Work out the finished part from the listing and answer in its coordinate system (mm). A direction names the side the tool comes from. Coordinates: 2 decimals unless noted, no trailing zeros. Write each loop counter-clockwise with the first axis right and the second up, starting at its lowest first coordinate (ties: lowest second). Pieces come first, ordered by that corner, then holes. Notation, with made-up numbers: (25.25, 1) - (59.25, 1) arc R33 cw to (59.25, 30) - close; hole circle Ø10 at (32.25, 23.5). An arc over 180 degrees is marked (long way). Use one line per item in the form item = value. Start each with the question number.
Item 1: A cutting plane is placed at C-C (z = 1.7). Give the number of separate pieces and of enclosed holes in the cut face, then the cut area to 3 significant figures.
Item 2: A cutting plane is placed at A-A (x = 25). Write down the section's boundary in (y, z).
Item 3: Consider probe 1 along Y at (x, z) = (25, 2.45); probe 2 along X at (y, z) = (5.25, 1.85); probe 3 along X at (y, z) = (7, 2). Determine where each line is inside the solid, lowest interval first.
Item 4: A cutting plane is placed at D-D (y = 12). Write down the section's boundary in (x, z), then the cut area to 3 significant figures.
Item 5: Given pin 1 (1.4 mm diameter, centred on x = 0, z = 1.5, fed in from -Y); pin 2 (2.5 mm diameter, centred on x = -25, y = 4, fed in from +Z); pin 3 (1.5 mm diameter, centred on y = 7.5, z = 2.5, fed in from -X), each flat-ended and moving along its own axis, determine where each tip first touches the part or whether it passes through.
Item 6: For faces 1 (the flat face through (0, 9, 0.6)), 2 (the cylindrical face through (29, 4, 1)), 3 (the cylindrical face through (8.416, 9.866, 2.14)), determine the directions among +Z, -Z, +X, -X, +Y, -Y from which every point of the face is accessible in a straight line to the end or side of a thin tool.
Item 7: A cutting plane is placed at B-B (y = 4). Write down the section's boundary in (x, z).
from build123d import *

# Parameters (mm, degrees)
F0_R         = 2.1
F1_DEPTH     = 3
F3_SIZE2     = 2
F3_SIZE      = 2
F4_T4_DEPTH  = 11.7592419794
F4_T10_DEPTH = 11.7592419794


# Not quite as in the source:
# - a fillet or chamfer that OpenCascade refuses, or shapes differently, is made with other operations: its cross-section is extruded or revolved along the edge and cut away or added


with BuildPart() as f1:
    # F0 (on Top) → F1 (new body)
    with BuildSketch(Plane.XY):
        with BuildLine():
            Line((0, 9), (0, 14.5))
            Line((0, 14.5), (-12, 14.5))
            Line((-12, 14.5), (-23.2738011309, 7.6083566155))
            ThreePointArc((-23.2738011309, 7.6083566155), (-28.988394733, 3.6955210129), (-22.746064478, 0.6954917669))
            Line((-22.746064478, 0.6954917669), (-10.5707757175, 9))
            Line((-10.5707757175, 9), (0, 9))
        make_face()
        with Locations((-25, 4)):
            Circle(F0_R, mode=Mode.SUBTRACT)
    extrude(amount=F1_DEPTH)

    # F2: F1 across plane


with BuildPart() as f1_1:
    add(f1.part)
    add(f1.part.mirror(Plane.YZ))

    # F3
    f3_edges = [f1_1.edges().sort_by_distance(p)[0] for p in [
        (0, 9, 3),
    ]]
    chamfer(f3_edges, length=F3_SIZE, length2=F3_SIZE2)

    # F4: fillet of radius 3 on 2 edges, made by hand


with BuildPart() as f4_tool2:
    # F4_s3 → F4_t4 (new body)
    with BuildSketch(Plane(origin=(-3.7553101229, 2.5614180039, 2.5614180039), x_dir=(0.5634838805, 0.8261270583, 0), z_dir=(0.7197293509, -0.4909122434, -0.4909122434))):
        with BuildLine():
            ThreePointArc((12.1440853808, 1.7707824696), (13.0615715756, 2.8377506524), (13.3916052457, 4.2056979457))
            Line((13.3916052457, 4.2056979457), (13.3916052457, 2.6686591321))
            Line((13.3916052457, 2.6686591321), (12.1440853808, 1.7707824696))
        make_face()
    extrude(amount=F4_T4_DEPTH)

    split(bisect_by=Plane.XY.offset(3), keep=Keep.BOTTOM)

    split(bisect_by=Plane.XZ.offset(-9), keep=Keep.BOTTOM)


with BuildPart() as f1_2:
    add(f1_1.part)

    # F4_t1: union F4_tool2
    add(f4_tool2.part)


with BuildPart() as f4_tool8:
    # F4_s9 → F4_t10 (new body)
    with BuildSketch(Plane(origin=(3.7553101229, 2.5614180039, 2.5614180039), x_dir=(0.5634838805, -0.8261270583, 0), z_dir=(-0.7197293509, -0.4909122434, -0.4909122434))):
        with BuildLine():
            ThreePointArc((-13.3916052457, 4.2056979457), (-13.0615715756, 2.8377506524), (-12.1440853808, 1.7707824696))
            Line((-12.1440853808, 1.7707824696), (-13.3916052457, 2.6686591321))
            Line((-13.3916052457, 2.6686591321), (-13.3916052457, 4.2056979457))
        make_face()
    extrude(amount=F4_T10_DEPTH)

    split(bisect_by=Plane.XY.offset(3), keep=Keep.BOTTOM)

    split(bisect_by=Plane.XZ.offset(-9), keep=Keep.BOTTOM)


with BuildPart() as f1_3:
    add(f1_2.part)

    # F4_t7: union F4_tool8
    add(f4_tool8.part)


solid = f1_3.part
Answer:
q1.separate_pieces = 1
q1.enclosed_holes = 2
q1.area = 325 mm²
q2.outline = (0, 0) - (1.9, 0) - (1.9, 3) - (0, 3) - close; (6.1, 0) - (8, 0) - (8, 3) - (6.1, 3) - close
q3.probe_1 = 0 to 1.9, 6.1 to 8
q3.probe_2 = -28.8 to -26.69, -23.31 to -16.07, 16.07 to 23.31, 26.69 to 28.8
q3.probe_3 = -27.65 to -13.5, 13.5 to 27.65
q4.outline = (-16.09, 0) - (16.09, 0) - (16.09, 3) - (-16.09, 3) - close
q4.area = 96.5 mm²
q5.pin_1 = 9
q5.pin_2 = through
q5.pin_3 = -27.9
q6.face_1 = +Z, -Z, -Y
q6.face_2 = +Z, -Z
q6.face_3 = +Z, -Y
q7.outline = (-29, 0) - (-27.1, 0) - (-27.1, 3) - (-29, 3) - close; (-22.9, 0) - (-17.9, 0) - (-17.9, 3) - (-22.9, 3) - close; (17.9, 0) - (22.9, 0) - (22.9, 3) - (17.9, 3) - close; (27.1, 0) - (29, 0) - (29, 3) - (27.1, 3) - close
